Verification items for the finished model (mm, model axes). Give positions to 0.01 mm unless a question says otherwise; leave off trailing zeros. Loops run counter-clockwise (first coordinate to the right, second up) from the corner with the lowest first, then second, coordinate; pieces in that order, holes last. Notation, with made-up numbers: M 46.25,-3 L 93.25,-3 A18 cw 93.25,32 Z; hole C 63,17.5 d1. An arc over 180 degrees is marked long. Use a Markdown table: item, result.
from build123d import *

# Parameters (mm, degrees)
CROQUIS1_R              = 2.5
SALIENTE_EXTRUIR1_DEPTH = 8.5


with BuildPart() as part:
    # Croquis1 → Saliente-Extruir1 (new, symmetric)
    with BuildSketch(Plane(origin=(0, 0, 0), x_dir=(0, 0, -1), z_dir=(1, 0, 0))):
        with BuildLine():
            Line((0, 7.5), (-17, 7.5))
            ThreePointArc((-17, 7.5), (-24.5, 0), (-17, -7.5))
            Line((-17, -7.5), (0, -7.5))
            ThreePointArc((0, -7.5), (7.5, 0), (0, 7.5))
        make_face()
        Circle(CROQUIS1_R, mode=Mode.SUBTRACT)
    extrude(amount=SALIENTE_EXTRUIR1_DEPTH, both=True)


solid = part.part
(1) Gauge pin test, flat end, axial feed: P1, Ø6, axis at x = -1, y = -5.5, coming from the -Z side. Record the tip position at first contact, or that the pin passes through.
Results below:
| item | result |
|---|---|
| P1 | z = -7.07 |
(2) Cross-section at A-A on z = 2. Record the cut outline in (x, y).
Results below:
| item | result |
|---|---|
| outline | M -8.5,-7.5 L 8.5,-7.5 L 8.5,-1.5 L -8.5,-1.5 Z; M -8.5,1.5 L 8.5,1.5 L 8.5,7.5 L -8.5,7.5 Z |
(3) Cross-section at B-B on y = 0. Record the cut outline in (x, z).
Results below:
| item | result |
|---|---|
| outline | M -8.5,-7.5 L 8.5,-7.5 L 8.5,-2.5 L -8.5,-2.5 Z; M -8.5,2.5 L 8.5,2.5 L 8.5,24.5 L -8.5,24.5 Z |
(4) Cross-section at D-D on z = -4.5. Record the cut outline in (x, y).
Results below:
| item | result |
|---|---|
| outline | M -8.5,-6 L 8.5,-6 L 8.5,6 L -8.5,6 Z |
(5) Material ranges on line 1 (Y direction, x = 0.25, z = 0); line 2 (Z direction, x = -2, y = 1.5); line 3 (Z direction, x = 6.5, y = 1), recorded low to high.
Results below:
| item | result |
|---|---|
| line 1 | -7.5 to -2.5, 2.5 to 7.5 |
| line 2 | -7.35 to -2, 2 to 24.35 |
| line 3 | -7.43 to -2.29, 2.29 to 24.43 |
(6) Draft check along Y on faces 1 (the cylindrical face through (-0.12, -2.44, 0.54)), 2 (the flat face through (0, -7.5, 9)), 3 (the flat face through (-8.5, 0, 9)), 4 (the flat face through (0, 7.5, 8)). Enter one of: +Y half, -Y half, draft (parallel to the pull), parting line (faces both ways), or undercut.
Results below:
| item | result |
|---|---|
| face 1 | undercut |
| face 2 | -Y half |
| face 3 | draft |
| face 4 | +Y half |
(7) Cross-section at C-C on x = 3.5. Record the cut outline in (y, z), then the cut area to 3 significant figures.
Results below:
| item | result |
|---|---|
| outline | M -7.5,0 A7.5 ccw 7.5,0 L 7.5,17 A7.5 ccw -7.5,17 Z; hole C 0,0 d5 |
| area | 412 mm^2 |
